Design review of the part shown in the three views and the two pictorial views. Dimensions are in mm from the part's minimum x, y and z. A direction names the side the tool comes from. Round coordinates to 2 decimals unless told otherwise and drop trailing zeros. Order: outer loops, then holes, each group sorted by start corner. A loop starts at its lowest first (then second) coordinate and runs counter-clockwise, first axis right, second up.
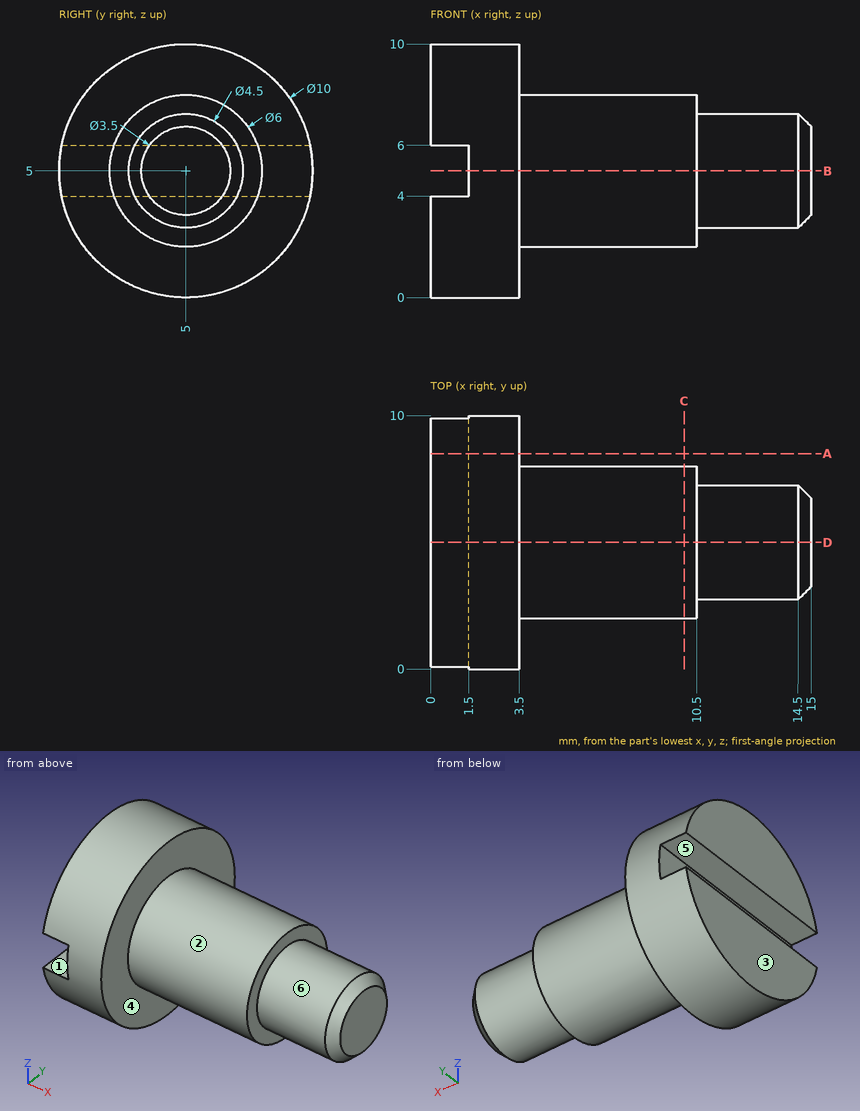
1) Clearance check with flat-ended pins moving along their axes: P1, Ø0.8, axis at x = 0.5, y = 6, coming from the +Z side; P2, Ø4, axis at x = 10, z = 6, coming from the -Y side; P3, Ø1, axis at x = 8, y = 6.5, coming from the -Z side. State where each tip first meets the part, or that it passes through.
Results:
P1: stops at z = 9.96
P2: stops at y = 2
P3: stops at z = 2.17
2) To check wall thickness, follow line 1 along X through (y, z) = (4, 9.75); line 2 along X through (y, z) = (7.5, 3.5); line 3 along Z through (x, y) = (2, 4). State the ranges of each line that lie inside material, in increasing order.
Results:
line 1: x = 0 to 3.5
line 2: x = 0 to 10.5
line 3: z = 0.1 to 9.9
3) Take a section at D-D on y = 5. Give the boundary of the cut face in (x, z).
Results:
outline: (0, 0) - (3.5, 0) - (3.5, 2) - (10.5, 2) - (10.5, 2.75) - (14.5, 2.75) - (15, 3.25) - (15, 6.75) - (14.5, 7.25) - (10.5, 7.25) - (10.5, 8) - (3.5, 8) - (3.5, 10) - (0, 10) - (0, 6) - (1.5, 6) - (1.5, 4) - (0, 4) - close
4) Take a section at C-C on x = 10. Give the boundary of the cut face in (y, z).
Results:
outline: circle Ø6 at (5, 5)
5) For the marked faces 1, 2 and 3, list the 3-axis set-ups (+Z, -Z, +X, -X, +Y, -Y) from which the entire face can be reached by the end or side of a thin tool; tool diameter is ignored.
Results:
face 1: -X, +Y, -Y
face 2: +X
face 3: +Z, -Z, -X, +Y, -Y
6) The part is to be moulded in two halves that separate along Z. For the marked faces 4, 5 and 6, say which applies: released by +Z, released by -Z, zero draft, split by the parting line, or undercut.
Results:
face 4: zero draft
face 5: undercut
face 6: split by the parting line
7) Take a section at B-B on z = 5. Give the boundary of the cut face in (x, y).
Results:
outline: (1.5, 0) - (3.5, 0) - (3.5, 2) - (10.5, 2) - (10.5, 2.75) - (14.5, 2.75) - (15, 3.25) - (15, 6.75) - (14.5, 7.25) - (10.5, 7.25) - (10.5, 8) - (3.5, 8) - (3.5, 10) - (1.5, 10) - close
8) Take a section at A-A on y = 8.5. Give the boundary of the cut face in (x, z), plus the area to 3 significant figures.
Results:
outline: (0, 1.43) - (3.5, 1.43) - (3.5, 8.57) - (0, 8.57) - (0, 6) - (1.5, 6) - (1.5, 4) - (0, 4) - close
area: 22.0 mm2
